Build history of the part. All positions in model axes, mm. Face numbers are marked on the shaded views. A direction names the side the tool comes from. Round coordinates to 2 decimals unless told otherwise and drop trailing zeros. Loops run counter-clockwise (first coordinate to the right, second up) from the corner with the lowest first, then second, coordinate; pieces in that order, holes last. Notation, with made-up numbers: M 17,53.5 L 41,53.5 A19 cw 41,60.5 Z; hole C -10.5,37.5 d5. An arc over 180 degrees is marked long. One line per item, written item: value.
```python
from build123d import *

# Parameters (mm, degrees)
SKETCH_3_W           = 50
SKETCH_3_H           = 50
EXTRUDE_1_DEPTH      = 10
FILLET_7_R           = 6
FILLET_8_R           = 6
FILLET_9_R           = 6
FILLET_10_R          = 6
SKETCH_4_R           = 3
CUT_EXTRUDE_1_DEPTH  = 37.742346142
SKETCH_6_R           = 3
CUT_EXTRUDE_14_DEPTH = 37.742346142
SKETCH_7_R           = 3
CUT_EXTRUDE_15_DEPTH = 37.742346142
SKETCH_8_R           = 3
CUT_EXTRUDE_16_DEPTH = 37.742346142
SKETCH_9_R           = 18
EXTRUDE_4_DEPTH      = 51
SKETCH_12_R          = 8
EXTRUDE_5_DEPTH      = 31
SKETCH_10_R          = 14
CUT_EXTRUDE_17_DEPTH = 65.707032123


with BuildPart() as part:
    # 草图3 → 凸台-拉伸1 (new body)
    with BuildSketch(Plane(origin=(0, 0, 0), x_dir=(1, 0, 0), z_dir=(0, 1, 0))):
        Rectangle(SKETCH_3_W, SKETCH_3_H)
    extrude(amount=EXTRUDE_1_DEPTH)

    # 圆角7
    fillet_7_edges = [part.edges().sort_by_distance(p)[0] for p in [
        (-25, 5, -25),
    ]]
    fillet(fillet_7_edges, radius=FILLET_7_R)

    # 圆角8
    fillet_8_edges = [part.edges().sort_by_distance(p)[0] for p in [
        (-25, 5, 25),
    ]]
    fillet(fillet_8_edges, radius=FILLET_8_R)

    # 圆角9
    fillet_9_edges = [part.edges().sort_by_distance(p)[0] for p in [
        (25, 5, 25),
    ]]
    fillet(fillet_9_edges, radius=FILLET_9_R)

    # 圆角10
    fillet_10_edges = [part.edges().sort_by_distance(p)[0] for p in [
        (25, 5, -25),
    ]]
    fillet(fillet_10_edges, radius=FILLET_10_R)

    # 草图4 → 切除-拉伸1 (cut, through all)
    with BuildSketch(Plane(origin=(0, 10, 0), x_dir=(1, 0, 0), z_dir=(0, 1, 0))):
        with Locations(Location((-19, -19, 0), (0, 0, 270))):
            Circle(SKETCH_4_R)
    extrude(amount=-CUT_EXTRUDE_1_DEPTH, mode=Mode.SUBTRACT)

    # 草图6 → 切除-拉伸14 (cut, through all)
    with BuildSketch(Plane(origin=(0, 10, 0), x_dir=(1, 0, 0), z_dir=(0, 1, 0))):
        with Locations(Location((-19, 19, 0), (0, 0, 270))):
            Circle(SKETCH_6_R)
    extrude(amount=-CUT_EXTRUDE_14_DEPTH, mode=Mode.SUBTRACT)

    # 草图7 → 切除-拉伸15 (cut, through all)
    with BuildSketch(Plane(origin=(0, 10, 0), x_dir=(1, 0, 0), z_dir=(0, 1, 0))):
        with Locations(Location((19, 19, 0), (0, 0, 270))):
            Circle(SKETCH_7_R)
    extrude(amount=-CUT_EXTRUDE_15_DEPTH, mode=Mode.SUBTRACT)

    # 草图8 → 切除-拉伸16 (cut, through all)
    with BuildSketch(Plane(origin=(0, 10, 0), x_dir=(1, 0, 0), z_dir=(0, 1, 0))):
        with Locations(Location((19, -19, 0), (0, 0, 270))):
            Circle(SKETCH_8_R)
    extrude(amount=-CUT_EXTRUDE_16_DEPTH, mode=Mode.SUBTRACT)

    # 草图9 → 凸台-拉伸4 (add)
    with BuildSketch(Plane(origin=(0, 0, 0), x_dir=(1, 0, 0), z_dir=(0, 1, 0))):
        with Locations(Location((0, 0, 0), (0, 0, 90))):
            Circle(SKETCH_9_R)
    extrude(amount=EXTRUDE_4_DEPTH)

    # 草图12 → 凸台-拉伸5 (add)
    with BuildSketch(Plane(origin=(0, 0, 0), x_dir=(0, 0, -1), z_dir=(1, 0, 0))):
        with Locations(Location((0, 26, 0), (0, 0, 180))):
            Circle(SKETCH_12_R)
    extrude(amount=EXTRUDE_5_DEPTH)

    # 草图10 → 切除-拉伸17 (cut, through all)
    with BuildSketch(Plane(origin=(0, 51, 0), x_dir=(1, 0, 0), z_dir=(0, 1, 0))):
        with Locations(Location((0, 0, 0), (0, 0, 270))):
            Circle(SKETCH_10_R)
    extrude(amount=-CUT_EXTRUDE_17_DEPTH, mode=Mode.SUBTRACT)


solid = part.part
```
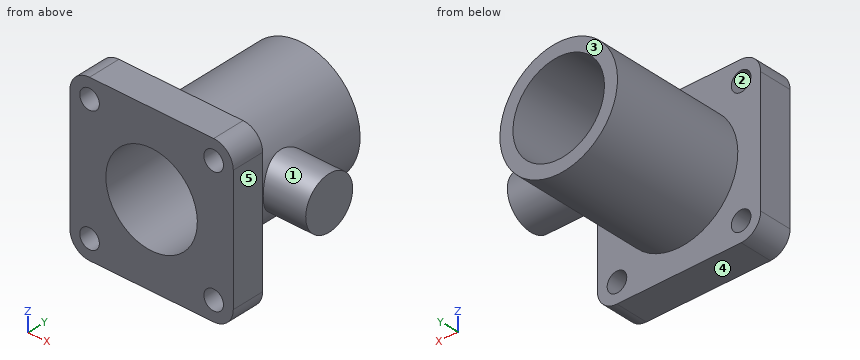
Item 1: Slice it at C-C, the plane y = 46.5. Give the cut face in (x, z), and give its area (3 significant figures).
Check values:
outline: C 0,0 d36; hole C 0,0 d28
area: 402 mm2
Item 2: Wall check: line 1 along X through (y, z) = (4.25, -19); line 2 along X through (y, z) = (39.5, 0); line 3 along Z through (x, y) = (7, 23.5). Give the ranges that are in metal, low to high.
Check values:
line 1: x = -25 to -22, -16 to 16, 22 to 25
line 2: x = -18 to -14, 14 to 18
line 3: z = -16.58 to -12.12, 12.12 to 16.58
Item 3: Drop flat-ended pins along their axis: P1, Ø4, axis at y = 22.5, z = -5.5, coming from the -X side; P2, Ø9.5, axis at x = 19, z = 19, coming from the +Y side; P3, Ø4, axis at y = 7.5, z = 8, coming from the +X side. Give the stop position or say it passes through.
Check values:
P1: stops at x = -17.66
P2: stops at y = 10
P3: stops at x = 25
Item 4: Which spindle directions (+Z, -Z, +X, -X, +Y, -Y) get a long thin tool onto all of the face, cutting with end or side? Do the marked faces 4 and 5. Say none if no direction does.
Check values:
face 4: -Z, +X, -X, +Y, -Y
face 5: +Z, -Z, +X, -Y
Item 5: Slice it at D-D, the plane z = 10. Give the cut face in (x, y).
Check values:
outline: M -25,0 L -9.8,0 L -9.8,51 L -14.97,51 L -14.97,10 L -25,10 Z; M 9.8,0 L 25,0 L 25,10 L 14.97,10 L 14.97,51 L 9.8,51 Z
Item 6: Pull direction Y, two halves, no side cores. Call the marked faces 1, 2 and 3: pulls with the +Y half, pulls with the -Y half, needs draft (parallel to the pull), parting line crosses it, or undercut.
Check values:
face 1: undercut
face 2: needs draft
face 3: pulls with the +Y half
Item 7: Slice it at A-A, the plane z = 0. Give the cut face in (x, y).
Check values:
outline: M -25,0 L -14,0 L -14,51 L -18,51 L -18,10 L -25,10 Z; M 14,0 L 25,0 L 25,10 L 18,10 L 18,18 L 31,18 L 31,34 L 18,34 L 18,51 L 14,51 Z
Item 8: Slice it at B-B, the plane x = -12.5. Give the cut face in (y, z).
Check values:
outline: M 0,-25 L 10,-25 L 10,-12.95 L 51,-12.95 L 51,-6.3 L 0,-6.3 Z; M 0,6.3 L 51,6.3 L 51,12.95 L 10,12.95 L 10,25 L 0,25 Z
